Part model, mm, in its own coordinate system. A direction names the side the tool comes from. Coordinates: 2 decimals unless noted, no trailing zeros. Loops run counter-clockwise (first coordinate to the right, second up) from the corner with the lowest first, then second, coordinate; pieces in that order, holes last. Notation, with made-up numbers: (-16.5, -9.5) -> (0.5, -9.5) arc R7 ccw to (0.5, -3.5) -> close; hole circle Ø8 at (62.25, -11.5). An arc over 180 degrees is marked (long way). One line per question, with ' | ' between items. Start each with the question number.
1) Cut at A-A (y = 21). List the corners of the cut face in (x, z), plus the area to 3 significant figures.
2) Drop flat-ended pins along their axis: pin 1 (10 mm diameter, centred on x = 5.5, y = 26, fed in from +Z); pin 2 (2.5 mm diameter, centred on y = 20, z = 5.5, fed in from -X); pin 3 (2.5 mm diameter, centred on y = 13, z = 5, fed in from +X). Give the stop position or say it passes through.
3) Cut at C-C (x = -26). List the corners of the cut face in (y, z).
4) 3-axis set-ups, long thin cutter, end or side, ignore diameter. For faces 1 (the face through (-17.78, 0, 11)), 2 (the face through (-1, 1, 0)): which of +Z, -Z, +X, -X, +Y, -Y reach the whole face in a straight line?
5) Cut at B-B (x = -40). List the corners of the cut face in (y, z).
6) Probe L1, parallel to Y at x = 36, z = 9; L2, parallel to Y at x = -31.5, z = 7; L3, parallel to X at y = -2, z = 14. List the from-to ranges inside material, lowest first. Write a range as from..to.
7) Two-plate mould, pull along Y, no slides. Class faces 3 (the face through (51.59, -0.21, 12.37)), 4 (the face through (-1, -50.8, 9)), 5 (the face through (33, -49.212, 10)), 6 (the face through (-16.828, -37, 10)): released by +Y, released by -Y, zero draft, split by the parting line, or undercut.
from build123d import *

# Parameters (mm, degrees)
F0_W     = 101.6
F0_H     = 101.6
F1_DEPTH = 1.5875
F2_W     = 101.6
F2_H     = 101.6
F2_W_2   = 98.425
F2_H_2   = 98.425
F3_DEPTH = 16.1925
F4_W     = 25.4
F4_H     = 1.5875
F4_W_2   = 1.5875
F4_H_2   = 25.4
F5_DEPTH = 16.1925
F6_W     = 12.7
F6_H     = 5.08
F6_W_2   = 5.08
F6_H_2   = 12.7
F7_DEPTH = 6.35
F8_R     = 1.5875
F9_DEPTH = 2.54
F11_R    = 0.94615


with BuildPart() as f1:
    # F0 (on Top) → F1 (new body)
    with BuildSketch(Plane.XY):
        Rectangle(F0_W, F0_H)
    extrude(amount=F1_DEPTH)

    # F2 (on face) → F3 (join)
    with BuildSketch(Plane.XY.offset(1.5875)):
        Rectangle(F2_W, F2_H)
        Rectangle(F2_W_2, F2_H_2, mode=Mode.SUBTRACT)
    extrude(amount=F3_DEPTH)

    # F4 (on face) → F5 (join, through all)
    with BuildSketch(Plane.XY.offset(1.5875)):
        with Locations((-36.5125, -16.03375)):
            Rectangle(F4_W, F4_H)
        with Locations((36.5125, -16.03375)):
            Rectangle(F4_W, F4_H)
        with Locations((-36.5125, 16.03375)):
            Rectangle(F4_W, F4_H)
        with Locations((36.5125, 16.03375)):
            Rectangle(F4_W, F4_H)
        with Locations((16.03375, 36.5125)):
            Rectangle(F4_W_2, F4_H_2)
        with Locations((-16.03375, 36.5125)):
            Rectangle(F4_W_2, F4_H_2)
        with Locations((-16.03375, -36.5125)):
            Rectangle(F4_W_2, F4_H_2)
        with Locations((16.03375, -36.5125)):
            Rectangle(F4_W_2, F4_H_2)
        with Locations((0, 16.98625)):
            Rectangle(F4_W, F4_H)
        with Locations((0, -16.98625)):
            Rectangle(F4_W, F4_H)
        with Locations((-16.98625, 0)):
            Rectangle(F4_W_2, F4_H_2)
        with Locations((16.98625, 0)):
            Rectangle(F4_W_2, F4_H_2)
    extrude(amount=F5_DEPTH)

    # F6 (on face) → F7 (join)
    with BuildSketch(Plane.XY.offset(1.5875)):
        with Locations((-36.5125, 12.7)):
            Rectangle(F6_W, F6_H)
        with Locations((-36.5125, -12.7)):
            Rectangle(F6_W, F6_H)
        with Locations((-12.7, 36.5125)):
            Rectangle(F6_W_2, F6_H_2)
        with Locations((12.7, 36.5125)):
            Rectangle(F6_W_2, F6_H_2)
        with Locations((36.5125, 12.7)):
            Rectangle(F6_W, F6_H)
        with Locations((36.5125, -12.7)):
            Rectangle(F6_W, F6_H)
        with Locations((12.7, -36.5125)):
            Rectangle(F6_W_2, F6_H_2)
        with Locations((-12.7, -36.5125)):
            Rectangle(F6_W_2, F6_H_2)
        with Locations((0, -20.32)):
            Rectangle(F6_W, F6_H)
        with Locations((20.32, 0)):
            Rectangle(F6_W_2, F6_H_2)
        with Locations((-20.32, 0)):
            Rectangle(F6_W_2, F6_H_2)
        with Locations((0, 20.32)):
            Rectangle(F6_W, F6_H)
    extrude(amount=F7_DEPTH)

    # F8 (on face) → F9 (join)
    with BuildSketch(Plane.YZ.offset(50.8)):
        with Locations((0, 10.795)):
            Circle(F8_R)
    extrude(amount=F9_DEPTH)

    # F10: F1 across plane


with BuildPart() as f1_1:
    add(f1.part)
    add(f1.part.mirror(Plane.YZ))

    # F11
    f11_edges = [f1_1.edges().sort_by_distance(p)[0] for p in [
        (-53.34, -1.5875, 10.795),
        (-50.8, -50.8, 8.89),
        (0, -50.8, 0),
        (50.8, -50.8, 8.89),
        (53.34, -1.5875, 10.795),
        (50.8, 0, 0),
        (0, 50.8, 0),
        (50.8, 50.8, 8.89),
        (-50.8, 0, 0),
        (-50.8, 50.8, 8.89),
    ]]
    fillet(f11_edges, radius=F11_R)


solid = f1_1.part
Reported:
1) outline: (-50.8, 0.95) arc R0.95 ccw to (-49.85, 0) -> (49.85, 0) arc R0.95 ccw to (50.8, 0.95) -> (50.8, 17.78) -> (49.21, 17.78) -> (49.21, 1.59) -> (6.35, 1.59) -> (6.35, 7.94) -> (-6.35, 7.94) -> (-6.35, 1.59) -> (-49.21, 1.59) -> (-49.21, 17.78) -> (-50.8, 17.78) -> close | area: 293 mm²
2) pin 1: stops at z = 7.94 | pin 2: stops at x = -50.8 | pin 3: stops at x = 50.8
3) outline: (-50.8, 0.95) arc R0.95 ccw to (-49.85, 0) -> (49.85, 0) arc R0.95 ccw to (50.8, 0.95) -> (50.8, 17.78) -> (49.21, 17.78) -> (49.21, 1.59) -> (16.83, 1.59) -> (16.83, 17.78) -> (15.24, 17.78) -> (15.24, 1.59) -> (-15.24, 1.59) -> (-15.24, 17.78) -> (-16.83, 17.78) -> (-16.83, 1.59) -> (-49.21, 1.59) -> (-49.21, 17.78) -> (-50.8, 17.78) -> close
4) face 1: +Z | face 2: -Z, +X, -X, +Y, -Y
5) outline: (-50.8, 0.95) arc R0.95 ccw to (-49.85, 0) -> (49.85, 0) arc R0.95 ccw to (50.8, 0.95) -> (50.8, 17.78) -> (49.21, 17.78) -> (49.21, 1.59) -> (16.83, 1.59) -> (16.83, 17.78) -> (15.24, 17.78) -> (15.24, 7.94) -> (10.16, 7.94) -> (10.16, 1.59) -> (-10.16, 1.59) -> (-10.16, 7.94) -> (-15.24, 7.94) -> (-15.24, 17.78) -> (-16.83, 17.78) -> (-16.83, 1.59) -> (-49.21, 1.59) -> (-49.21, 17.78) -> (-50.8, 17.78) -> close
6) L1: y = -50.8..-49.21, -16.83..-15.24, 15.24..16.83, 49.21..50.8 | L2: y = -50.8..-49.21, -16.83..-10.16, 10.16..16.83, 49.21..50.8 | L3: x = -50.8..-49.21, -17.78..-16.19, 16.19..17.78, 49.21..50.8
7) face 3: split by the parting line | face 4: released by -Y | face 5: undercut | face 6: undercut
